Source: CAD feature listing. Evaluate the final solid. Frame: model axes, mm. Face numbers are marked on the shaded views. A direction names the side the tool comes from. Give positions to 0.01 mm unless a question says otherwise; leave off trailing zeros. Order: outer loops, then holes, each group sorted by start corner. A loop starts at its lowest first (then second) coordinate and runs counter-clockwise, first axis right, second up.
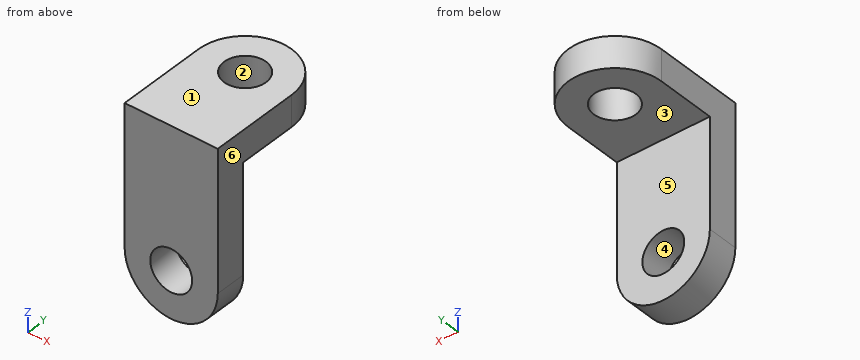
```python
from build123d import *

# Parameters (mm, degrees)
ESQUISSE1_W             = 15
ESQUISSE1_H             = 30
BOSS_EXTRU_1_DEPTH      = 5
ESQUISSE2_W             = 15
ESQUISSE2_H             = 5
BOSS_EXTRU_2_DEPTH      = 17
CONG_1_RADIUS           = 7.5
CONG_1_LENGTH           = 5
CONG_3_RADIUS           = 7.5
CONG_3_LENGTH           = 5
ESQUISSE3_R             = 3.375
ENL_V_MAT_EXTRU_1_DEPTH = 10
ESQUISSE4_R             = 3.375
ENL_V_MAT_EXTRU_2_DEPTH = 10


with BuildPart() as part:
    # Esquisse1 → Boss.-Extru.1 (new body)
    with BuildSketch(Plane(origin=(0, 0, 0), x_dir=(1, 0, 0), z_dir=(0, 1, 0))):
        with Locations((0, 1.739690722)):
            Rectangle(ESQUISSE1_W, ESQUISSE1_H)
    extrude(amount=BOSS_EXTRU_1_DEPTH)

    # Esquisse2 → Boss.-Extru.2 (add)
    with BuildSketch(Plane(origin=(0, 5, 0), x_dir=(1, 0, 0), z_dir=(0, 1, 0))):
        with Locations((0, -10.760309278)):
            Rectangle(ESQUISSE2_W, ESQUISSE2_H)
    extrude(amount=BOSS_EXTRU_2_DEPTH)

    # Congé1: full round fillet: the end face becomes a half cylinder, R = half its width
    cong_1_face = Plane((0, 2.5, -16.739690722), x_dir=(0, 1, 0), z_dir=(0, 0, -1))  # on the end face: x along it, z out of the body
    cong_1_slab = cong_1_face.offset(-CONG_1_RADIUS / 2) * Box(CONG_1_LENGTH, 2 * CONG_1_RADIUS, CONG_1_RADIUS, mode=Mode.PRIVATE)  # the body's end, R deep
    cong_1_round = Plane((0, 2.5, -9.239690722), x_dir=(0, 0, -1), z_dir=(0, 1, 0)) * Cylinder(CONG_1_RADIUS, CONG_1_LENGTH, mode=Mode.PRIVATE)  # its axis R under the face
    add(cong_1_slab - cong_1_round, mode=Mode.SUBTRACT)

    # Congé3: full round fillet: the end face becomes a half cylinder, R = half its width
    cong_3_face = Plane((0, 22, 10.760309278), x_dir=(0, 0, -1), z_dir=(0, 1, 0))  # on the end face: x along it, z out of the body
    cong_3_slab = cong_3_face.offset(-CONG_3_RADIUS / 2) * Box(CONG_3_LENGTH, 2 * CONG_3_RADIUS, CONG_3_RADIUS, mode=Mode.PRIVATE)  # the body's end, R deep
    cong_3_round = Plane((0, 14.5, 10.760309278), x_dir=(0, 1, 0), z_dir=(0, 0, -1)) * Cylinder(CONG_3_RADIUS, CONG_3_LENGTH, mode=Mode.PRIVATE)  # its axis R under the face
    add(cong_3_slab - cong_3_round, mode=Mode.SUBTRACT)

    # Esquisse3 → Enlèv. mat.-Extru.1 (cut)
    with BuildSketch(Plane(origin=(0, 5, 0), x_dir=(1, 0, 0), z_dir=(0, 1, 0))):
        with Locations(Location((0, 9.239690722, 0), (0, 0, 270))):
            Circle(ESQUISSE3_R)
    extrude(amount=-ENL_V_MAT_EXTRU_1_DEPTH, mode=Mode.SUBTRACT)

    # Esquisse4 → Enlèv. mat.-Extru.2 (cut)
    with BuildSketch(Plane(origin=(0, 0, 8.260309278), x_dir=(-1, 0, 0), z_dir=(0, 0, -1))):
        with Locations((0, 14.5)):
            Circle(ESQUISSE4_R)
    extrude(amount=-ENL_V_MAT_EXTRU_2_DEPTH, mode=Mode.SUBTRACT)


solid = part.part
```
1) Draft query along Z for the marked faces 1, 2, 3 and 4. Return one class per face: +Z half, -Z half, draft (parallel to the pull), parting line (faces both ways), or undercut.
Report:
face 1: +Z half
face 2: draft
face 3: -Z half
face 4: undercut
2) Pin query (flat end, axial travel): pin 1 (1.5 mm diameter, centred on x = 1.5, z = 0, fed in from +Y); pin 2 (4 mm diameter, centred on x = 4, y = 11.5, fed in from -Z). Return the tip coordinate at first contact, or that it passes through.
Report:
pin 1: stops at y = 5
pin 2: stops at z = 8.26
3) Section query D-D, the plane y = 1.5. Return the cut outline in (x, z) (3 decimals).
Report:
outline: (-7.5, -9.24) arc R7.5 ccw to (7.5, -9.24) - (7.5, 13.26) - (-7.5, 13.26) - close; hole circle Ø6.75 at (0, -9.24)
4) Reachability of the marked faces 5 and 6 from +Z, -Z, +X, -X, +Y, -Y: full face, straight path, thin tool, end or side. Return the list, or none.
Report:
face 5: -Z, +X, -X, +Y
face 6: +Z, -Z, +X, +Y, -Y
5) Section query A-A, the plane x = 0. Return the cut outline in (y, z) (3 decimals), and give its area (4 significant figures).
Report:
outline: (0, -16.74) - (5, -16.74) - (5, -12.615) - (0, -12.615) - close; (0, -5.865) - (5, -5.865) - (5, 8.26) - (11.125, 8.26) - (11.125, 13.26) - (0, 13.26) - close; (17.875, 8.26) - (22, 8.26) - (22, 13.26) - (17.875, 13.26) - close
area: 167.5 mm2
6) Material intervals for L1, parallel to Y at x = 0, z = 12.1 (3 decimals); L2, parallel to Z at x = 6, y = 5.5; L3, parallel to Y at x = -3.5, z = -8.5, sorted ascending.
Report:
L1: y = 0 to 11.125, 17.875 to 22
L2: z = 8.26 to 13.26
L3: y = 0 to 5
7) Section query B-B, the plane y = 16. Return the cut outline in (x, z).
Report:
outline: (-7.35, 8.26) - (-3.02, 8.26) - (-3.02, 13.26) - (-7.35, 13.26) - close; (3.02, 8.26) - (7.35, 8.26) - (7.35, 13.26) - (3.02, 13.26) - close
8) Section query C-C, the plane z = 10.25. Return the cut outline in (x, y) (3 decimals), and give its area (3 significant figures).
Report:
outline: (-7.5, 0) - (7.5, 0) - (7.5, 14.5) arc R7.5 ccw to (-7.5, 14.5) - close; hole circle Ø6.75 at (0, 14.5)
area: 270 mm2
